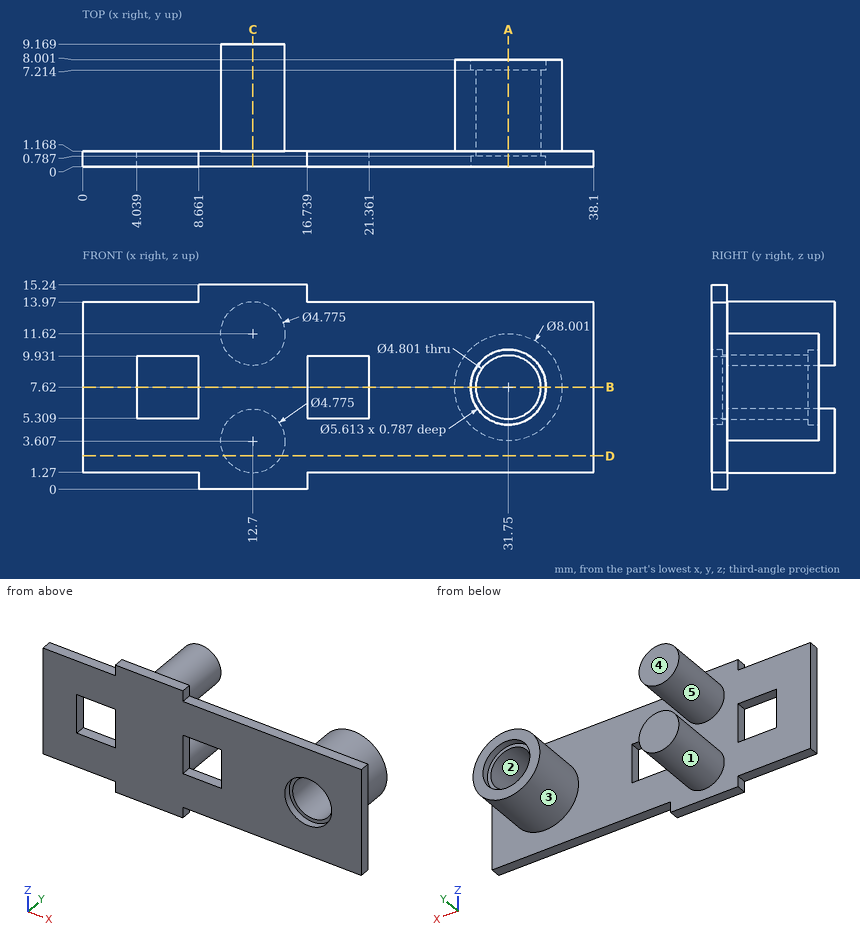
Geometry check sheet. Reference: drawing and pictorial views, mm from the part's lowest x, y, z. A direction names the side the tool comes from. Give positions to 0.01 mm unless a question says otherwise; leave off trailing zeros. Order: outer loops, then holes, each group sorted by start corner. A loop starts at its lowest first (then second) coordinate and runs counter-clockwise, first axis right, second up. Notation, with made-up numbers: (-14, -34.5) -> (21, -34.5) arc R32 ccw to (21, 3.5) -> close; hole circle Ø5 at (60, 86). An arc over 180 degrees is marked (long way). Use CSV: the item, a comma, the result in double quotes. Start each with the question number.
1) Mould release check, pull along Z, two halves, no side actions. Record for the marked faces 3, 4 and 5: released by +Z, released by -Z, zero draft, split by the parting line, or undercut.
2) Sectioned sample at A-A, the plane x = 31.75. Record the boundary of the cut face in (y, z).
3) Go/stop test with flat-tipped pins: P1, Ø1.3, axis at x = 7, y = 0.5, coming from the -Z side; P2, Ø3, axis at x = 33, z = 7, coming from the +Y side; P3, Ø1, axis at y = 3.5, z = 7, coming from the +X side. Record where each tip stops, or that it passes through.
4) Sectioned sample at D-D, the plane z = 2.5. Record the boundary of the cut face in (x, y) (1 decimal).
5) Sectioned sample at B-B, the plane z = 7.62. Record the boundary of the cut face in (x, y).
6) Set-up check for the marked faces 1 and 2: record each of +Z, -Z, +X, -X, +Y, -Y from which the full face is reachable in a straight line by a thin tool's end or side.
7) Sectioned sample at C-C, the plane x = 12.7. Record the boundary of the cut face in (y, z) (1 decimal).
8) Material ranges on line 1 (X direction, y = 7.7, z = 7.62); line 2 (Z direction, x = 31.75, y = 7.65); line 3 (Z direction, x = 31.75, y = 4.25), recorded low to high. Write a range as from..to.
Recorded:
1,face 3,"split by the parting line"
1,face 4,"zero draft"
1,face 5,"undercut"
2,outline,"(0, 1.27) -> (1.17, 1.27) -> (1.17, 3.62) -> (8, 3.62) -> (8, 4.81) -> (7.21, 4.81) -> (7.21, 5.22) -> (0.79, 5.22) -> (0.79, 4.81) -> (0, 4.81) -> close; (0, 10.43) -> (0.79, 10.43) -> (0.79, 10.02) -> (7.21, 10.02) -> (7.21, 10.43) -> (8, 10.43) -> (8, 11.62) -> (1.17, 11.62) -> (1.17, 13.97) -> (0, 13.97) -> close"
3,P1,"z = 1.27"
3,P2,"y = 8"
3,P3,"x = 35.75"
4,outline,"(0, 0) -> (38.1, 0) -> (38.1, 1.2) -> (14.8, 1.2) -> (14.8, 9.2) -> (10.6, 9.2) -> (10.6, 1.2) -> (0, 1.2) -> close"
5,outline,"(0, 0) -> (4.04, 0) -> (4.04, 1.17) -> (0, 1.17) -> close; (8.66, 0) -> (16.74, 0) -> (16.74, 1.17) -> (8.66, 1.17) -> close; (21.36, 0) -> (28.94, 0) -> (28.94, 0.79) -> (29.35, 0.79) -> (29.35, 7.21) -> (28.94, 7.21) -> (28.94, 8) -> (27.75, 8) -> (27.75, 1.17) -> (21.36, 1.17) -> close; (34.15, 0.79) -> (34.56, 0.79) -> (34.56, 0) -> (38.1, 0) -> (38.1, 1.17) -> (35.75, 1.17) -> (35.75, 8) -> (34.56, 8) -> (34.56, 7.21) -> (34.15, 7.21) -> close"
6,face 1,"+Y"
6,face 2,"+Y, -Y"
7,outline,"(0, 0) -> (1.2, 0) -> (1.2, 1.2) -> (9.2, 1.2) -> (9.2, 6) -> (1.2, 6) -> (1.2, 9.2) -> (9.2, 9.2) -> (9.2, 14) -> (1.2, 14) -> (1.2, 15.2) -> (0, 15.2) -> close"
8,line 1,"27.75..28.94, 34.56..35.75"
8,line 2,"3.62..4.81, 10.43..11.62"
8,line 3,"3.62..5.22, 10.02..11.62"
